Study the drawing (mm; zero at the part's minimum x, y, z) and answer. A direction names the side the tool comes from. Coordinates: 2 decimals unless noted, no trailing zeros. Order: outer loops, then holes, each group sorted by start corner. A loop starts at its lowest first (then second) coordinate and runs counter-clockwise, first axis right, second up. Notation, with made-up numbers: M 29.5,76 L 85.5,76 A23 ccw 85.5,94 Z; hole C 38.25,16 d6. An arc over 180 degrees is marked long. Put each result on its own line as item: value.
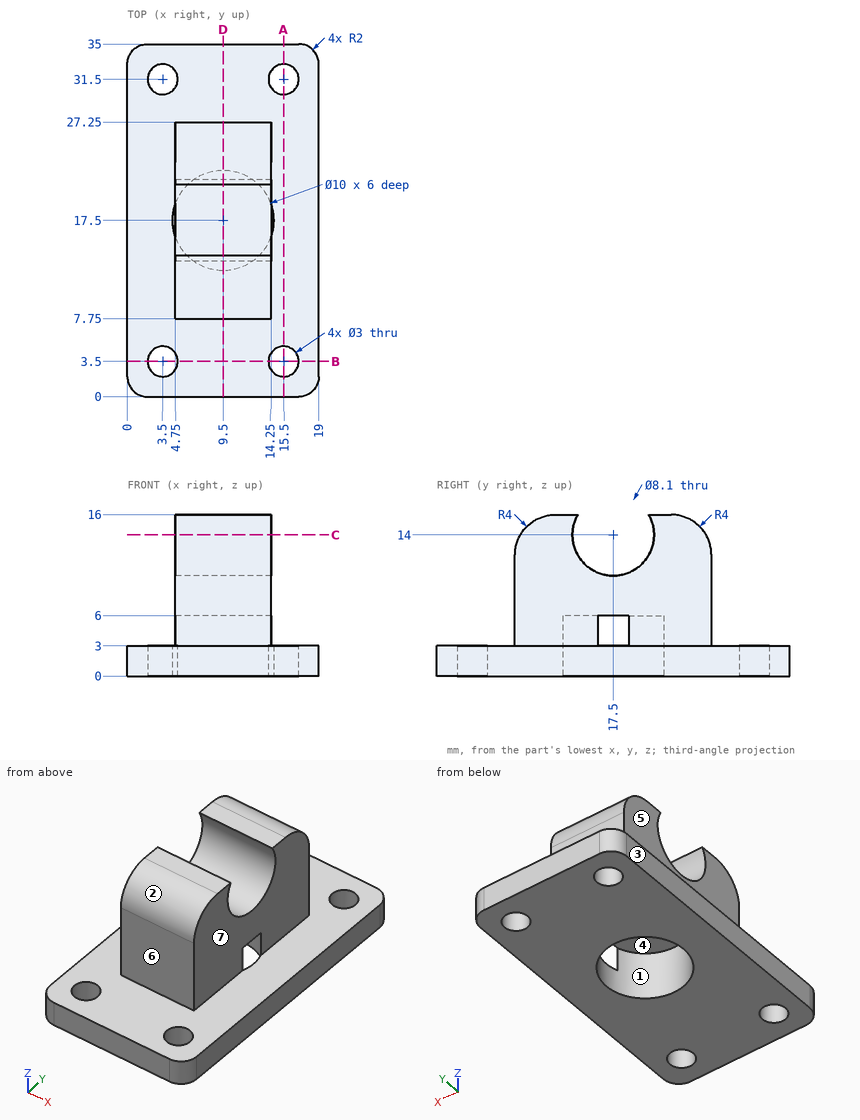
Q1. Find section A-A on x = 15.5. Write down the section's boundary in (y, z), plus the area to 3 significant figures.
Answers below:
outline: M 0,0 L 2,0 L 2,3 L 0,3 Z; M 5,0 L 30,0 L 30,3 L 5,3 Z; M 33,0 L 35,0 L 35,3 L 33,3 Z
area: 87.0 mm^2
Q2. A tool of negligible diameter and unlimited length cuts with its end or side. For the marked faces 4, 5, 6 and 7, from which of +Z, -Z, +X, -X, +Y, -Y can it reach the whole face along a straight path? Write none if from no direction.
Answers below:
face 4: -Z
face 5: +Z, -X, +Y, -Y
face 6: +Z, +X, -X, -Y
face 7: +Z, +X, +Y, -Y
Q3. Find section B-B on y = 3.5. Write down the section's boundary in (x, z).
Answers below:
outline: M 0,0 L 2,0 L 2,3 L 0,3 Z; M 5,0 L 14,0 L 14,3 L 5,3 Z; M 17,0 L 19,0 L 19,3 L 17,3 Z
Q4. Find section D-D on x = 9.5. Write down the section's boundary in (y, z).
Answers below:
outline: M 0,0 L 12.5,0 L 12.5,6 L 22.5,6 L 22.5,0 L 35,0 L 35,3 L 27.25,3 L 27.25,12 A4 ccw 23.25,16 L 21.02,16 A4.05 cw long 13.98,16 L 11.75,16 A4 ccw 7.75,12 L 7.75,3 L 0,3 Z
Q5. Find section C-C on z = 14. Write down the section's boundary in (x, y), plus the area to 3 significant figures.
Answers below:
outline: M 4.75,8.29 L 14.25,8.29 L 14.25,13.45 L 4.75,13.45 Z; M 4.75,21.55 L 14.25,21.55 L 14.25,26.71 L 4.75,26.71 Z
area: 98.1 mm^2
Q6. Given pin 1 (5 mm diameter, centred on x = 9, y = 17, fed in from -Z); pin 2 (2 mm diameter, centred on x = 5, z = 8.5, fed in from +Y); pin 3 (2 mm diameter, centred on x = 11, z = 14, fed in from -Y), each flat-ended and moving along its own axis, determine where each tip first touches the part or whether it passes through.
Answers below:
pin 1: stops at z = 6
pin 2: stops at y = 27.25
pin 3: stops at y = 7.88
Q7. Consider line 1 along Y through (x, z) = (3.5, 1.3); line 2 along Z through (x, y) = (11.25, 6); line 3 along X through (y, z) = (3, 1). Determine where each line is inside the solid, lowest interval first.
Answers below:
line 1: y = 0 to 2, 5 to 30, 33 to 35
line 2: z = 0 to 3
line 3: x = 0 to 2.09, 4.91 to 14.09, 16.91 to 19
Q8. For a pull along X with two mould halves and no side action, classify the marked faces 1, 2 and 3 as +X half, -X half, draft (parallel to the pull), parting line (faces both ways), or undercut.
Answers below:
face 1: undercut
face 2: draft
face 3: -X half
